Here's how the part is built. I have some questions about the finished solid (model axes, mm). A direction names the side the tool comes from. Round coordinates to 2 decimals unless told otherwise and drop trailing zeros. Order: outer loops, then holes, each group sorted by start corner. A loop starts at its lowest first (then second) coordinate and runs counter-clockwise, first axis right, second up. Notation, with made-up numbers: (60, 32) -> (86, 32) arc R19 cw to (86, 57) -> close; hole circle Ø3 at (24, 18). An arc over 180 degrees is marked (long way). Use a Markdown table: item, result. Add a question column.
from build123d import *

# Parameters (mm, degrees)
PAD_DEPTH    = 75
SKETCH001_R  = 2
POCKET_DEPTH = 9.001


with BuildPart() as part:
    # Sketch → Pad (new body, symmetric)
    with BuildSketch(Plane.XZ):
        Polygon((-3.5, 0), (-3.5, 8), (3.5, 8), (3.5, 0), (4.5, 0), (4.5, 9), (-4.5, 9), (-4.5, 0), align=None)
    extrude(amount=PAD_DEPTH, both=True)

    # Sketch001 → Pocket (cut, through all)
    with BuildSketch(Plane(origin=(4.5, 0, 0), x_dir=(0, 0, 1), z_dir=(1, 0, 0))):
        with Locations((4.5, 70)):
            Circle(SKETCH001_R)
        with Locations((4.5, -65)):
            Circle(SKETCH001_R)
        with Locations((4.5, -20)):
            Circle(SKETCH001_R)
    extrude(amount=-POCKET_DEPTH, mode=Mode.SUBTRACT)


solid = part.part
(1) I want a section at A-A on z = 4.5. State how many separate pieces and enclosed holes the cut face has, and give its area (3 significant figures).
(2) I want a section at B-B on y = -70. List the corners of the cut face in (x, z) for me.
(3) On a 3-axis mill with a long thin cutter (end or side, diameter ignored), from which of +Z, -Z, +X, -X, +Y, -Y can I reach the whole of each face in a straight line? I mean faces 4 (the flat face through (0, -1, 8)), 5 (the cylindrical face through (-3.993, 18.017, 4.24)). Say none if no direction works.
(4) I'm going to push flat-ended pins straight in: P1, Ø3, axis at y = 65, z = 4.5, coming from the -X side (1 decimal); P2, Ø4.5, axis at y = 65, z = 4.5, coming from the +X side; P3, Ø2, axis at x = 0, y = -33, coming from the -Z side. Where does each tip first touch, or does it pass through?
(5) If we mould it in two halves opening along Y, with no side actions, what happens to faces 1 (the flat face through (4.5, -1, 4)), 2 (the flat face through (-0.4, 75, 8.2)), 3 (the cylindrical face through (4.007, 18.017, 4.24))? For each: pulls with the +Y half, pulls with the -Y half, needs draft (parallel to the pull), parting line crosses it, or undercut.
(6) I want a section at C-C on y = -27.5. List the corners of the cut face in (x, z) for me, and give its area (3 significant figures).
(7) Please list where these lines run through material, in increasing order: probe 1 along Y at (x, z) = (-3.9, 4.5); probe 2 along X at (y, z) = (42.5, 4.5); probe 3 along Z at (x, y) = (-4.2, 65). Write a range as from..to.
Output:
| question | item | result |
|---|---|---|
| 1 | separate pieces | 8 |
| 1 | enclosed holes | 0 |
| 1 | area | 276 mm² |
| 2 | outline | (-4.5, 0) -> (-3.5, 0) -> (-3.5, 2.5) -> (-4.5, 2.5) -> close; (-4.5, 6.5) -> (-3.5, 6.5) -> (-3.5, 8) -> (3.5, 8) -> (3.5, 6.5) -> (4.5, 6.5) -> (4.5, 9) -> (-4.5, 9) -> close; (3.5, 0) -> (4.5, 0) -> (4.5, 2.5) -> (3.5, 2.5) -> close |
| 3 | face 4 | -Z, +Y, -Y |
| 3 | face 5 | +X, -X |
| 4 | P1 | through |
| 4 | P2 | x = 4.5 |
| 4 | P3 | z = 8 |
| 5 | face 1 | needs draft |
| 5 | face 2 | pulls with the +Y half |
| 5 | face 3 | undercut |
| 6 | outline | (-4.5, 0) -> (-3.5, 0) -> (-3.5, 8) -> (3.5, 8) -> (3.5, 0) -> (4.5, 0) -> (4.5, 9) -> (-4.5, 9) -> close |
| 6 | area | 25.0 mm² |
| 7 | probe 1 | -75..-72, -68..18, 22..63, 67..75 |
| 7 | probe 2 | -4.5..-3.5, 3.5..4.5 |
| 7 | probe 3 | 0..2.5, 6.5..9 |
